```python
from build123d import *

# Parameters (mm, degrees)
SKETCH1_W           = 124
SKETCH1_H           = 62
SKETCH1_R           = 6.5
SKETCH1_R_2         = 2
SKETCH1_W_2         = 22
SKETCH1_H_2         = 30
BOSS_EXTRUDE1_DEPTH = 2


with BuildPart() as part:
    # Sketch1 → Boss-Extrude1 (new body)
    with BuildSketch(Plane(origin=(0, 0, 0), x_dir=(1, 0, 0), z_dir=(0, 1, 0))):
        with Locations((14.5, 0)):
            Rectangle(SKETCH1_W, SKETCH1_H)
        with Locations((12.5, 11)):
            Circle(SKETCH1_R, mode=Mode.SUBTRACT)
        with Locations((12.5, -11)):
            Circle(SKETCH1_R, mode=Mode.SUBTRACT)
        with Locations((34.5, 11)):
            Circle(SKETCH1_R, mode=Mode.SUBTRACT)
        with Locations((34.5, -11)):
            Circle(SKETCH1_R, mode=Mode.SUBTRACT)
        with Locations((56.5, 0)):
            Circle(SKETCH1_R, mode=Mode.SUBTRACT)
        with Locations((-39.5, 23)):
            Circle(SKETCH1_R_2, mode=Mode.SUBTRACT)
        with Locations((68.5, 23)):
            Circle(SKETCH1_R_2, mode=Mode.SUBTRACT)
        with Locations((68.5, -23)):
            Circle(SKETCH1_R_2, mode=Mode.SUBTRACT)
        with Locations((-39.5, -23)):
            Circle(SKETCH1_R_2, mode=Mode.SUBTRACT)
        with Locations((-20, 0)):
            Rectangle(SKETCH1_W_2, SKETCH1_H_2, mode=Mode.SUBTRACT)
    extrude(amount=BOSS_EXTRUDE1_DEPTH)


solid = part.part
```
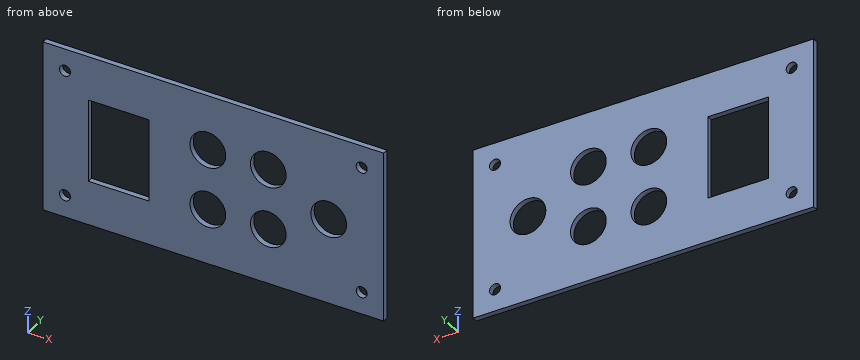
For this review, take the finished solid that the model builds, in its own axes (mm). Round coordinates to 2 decimals unless told otherwise and drop trailing zeros. Loops run counter-clockwise (first coordinate to the right, second up) from the corner with the lowest first, then second, coordinate; pieces in that order, holes last.
(1) We need section A-A (x = 12.5). Give the boundary of the cut face in (y, z), plus the area to 3 significant figures.
Returned:
outline: (0, -31) - (2, -31) - (2, -17.5) - (0, -17.5) - close; (0, -4.5) - (2, -4.5) - (2, 4.5) - (0, 4.5) - close; (0, 17.5) - (2, 17.5) - (2, 31) - (0, 31) - close
area: 72.0 mm2
(2) We need section B-B (x = 56.5). Give the boundary of the cut face in (y, z), plus the area to 3 significant figures.
Returned:
outline: (0, -31) - (2, -31) - (2, -6.5) - (0, -6.5) - close; (0, 6.5) - (2, 6.5) - (2, 31) - (0, 31) - close
area: 98.0 mm2
(3) Wall thickness on line 1 along Z through (x, y) = (68.5, 0.55); line 2 along X through (y, z) = (1.5, -11); line 3 along X through (y, z) = (1.2, -23): over which ranges is each line inside the solid? List them lowest first.
Returned:
line 1: z = -31 to -25, -21 to 21, 25 to 31
line 2: x = -47.5 to -31, -9 to 6, 19 to 28, 41 to 76.5
line 3: x = -47.5 to -41.5, -37.5 to 66.5, 70.5 to 76.5
(4) We need section C-C (z = 11). Give the boundary of the cut face in (x, y), plus the area to 3 significant figures.
Returned:
outline: (-47.5, 0) - (-31, 0) - (-31, 2) - (-47.5, 2) - close; (-9, 0) - (6, 0) - (6, 2) - (-9, 2) - close; (19, 0) - (28, 0) - (28, 2) - (19, 2) - close; (41, 0) - (76.5, 0) - (76.5, 2) - (41, 2) - close
area: 152 mm2
(5) We need section D-D (y = 1.55). State how many separate pieces and enclosed holes the cut face has, plus the area to 3 significant figures.
Returned:
separate pieces: 1
enclosed holes: 10
area: 6,310 mm2
